from build123d import *

# Parameters (mm, degrees)
BOX_W                = 35
BOX_H                = 35
BOX_DEPTH            = 18
BOX001_W             = 1.5217
BOX001_H             = 35
BOX001_DEPTH         = 16.5
BOX002_W             = 1.5217
BOX002_H             = 35
BOX002_DEPTH         = 16.5
BOX003_W             = 1.5217
BOX003_H             = 35
BOX003_DEPTH         = 16.5
BOX004_W             = 1.5217
BOX004_H             = 35
BOX004_DEPTH         = 16.5
BOX005_W             = 7.6087
BOX005_H             = 35
BOX005_DEPTH         = 16.5
BOX006_W             = 1.5217
BOX006_H             = 35
BOX006_DEPTH         = 16.5
BOX007_W             = 1.5217
BOX007_H             = 35
BOX007_DEPTH         = 16.5
BOX008_W             = 1.5217
BOX008_H             = 35
BOX008_DEPTH         = 16.5
BOX009_W             = 1.5217
BOX009_H             = 35
BOX009_DEPTH         = 16.5
BODY_PLACEMENT_ANGLE = 90


with BuildPart() as part:
    # Box → Box (join)
    with BuildSketch(Plane(origin=(-17.5, -17.5, 0), x_dir=(1, 0, 0), z_dir=(0, 0, 1))):
        with Locations((17.5, 17.5)):
            Rectangle(BOX_W, BOX_H)
    extrude(amount=BOX_DEPTH)

    # Box001 → Box001 (cut)
    with BuildSketch(Plane(origin=(-15.978, -17.5, 1.5), x_dir=(1, 0, 0), z_dir=(0, 0, 1))):
        with Locations((0.76085, 17.5)):
            Rectangle(BOX001_W, BOX001_H)
    extrude(amount=BOX001_DEPTH, mode=Mode.SUBTRACT)

    # Box002 → Box002 (cut)
    with BuildSketch(Plane(origin=(-12.9347, -17.5, 1.5), x_dir=(1, 0, 0), z_dir=(0, 0, 1))):
        with Locations((0.76085, 17.5)):
            Rectangle(BOX002_W, BOX002_H)
    extrude(amount=BOX002_DEPTH, mode=Mode.SUBTRACT)

    # Box003 → Box003 (cut)
    with BuildSketch(Plane(origin=(-9.891304, -17.5, 1.5), x_dir=(1, 0, 0), z_dir=(0, 0, 1))):
        with Locations((0.76085, 17.5)):
            Rectangle(BOX003_W, BOX003_H)
    extrude(amount=BOX003_DEPTH, mode=Mode.SUBTRACT)

    # Box004 → Box004 (cut)
    with BuildSketch(Plane(origin=(-6.84782, -17.5, 1.5), x_dir=(1, 0, 0), z_dir=(0, 0, 1))):
        with Locations((0.76085, 17.5)):
            Rectangle(BOX004_W, BOX004_H)
    extrude(amount=BOX004_DEPTH, mode=Mode.SUBTRACT)

    # Box005 → Box005 (cut)
    with BuildSketch(Plane(origin=(-3.80434, -17.5, 1.5), x_dir=(1, 0, 0), z_dir=(0, 0, 1))):
        with Locations((3.80435, 17.5)):
            Rectangle(BOX005_W, BOX005_H)
    extrude(amount=BOX005_DEPTH, mode=Mode.SUBTRACT)

    # Box006 → Box006 (cut)
    with BuildSketch(Plane(origin=(5.326088, -17.5, 1.5), x_dir=(1, 0, 0), z_dir=(0, 0, 1))):
        with Locations((0.76085, 17.5)):
            Rectangle(BOX006_W, BOX006_H)
    extrude(amount=BOX006_DEPTH, mode=Mode.SUBTRACT)

    # Box007 → Box007 (cut)
    with BuildSketch(Plane(origin=(8.369566, -17.5, 1.5), x_dir=(1, 0, 0), z_dir=(0, 0, 1))):
        with Locations((0.76085, 17.5)):
            Rectangle(BOX007_W, BOX007_H)
    extrude(amount=BOX007_DEPTH, mode=Mode.SUBTRACT)

    # Box008 → Box008 (cut)
    with BuildSketch(Plane(origin=(11.407644, -17.5, 1.5), x_dir=(1, 0, 0), z_dir=(0, 0, 1))):
        with Locations((0.76085, 17.5)):
            Rectangle(BOX008_W, BOX008_H)
    extrude(amount=BOX008_DEPTH, mode=Mode.SUBTRACT)

    # Box009 → Box009 (cut)
    with BuildSketch(Plane(origin=(14.456521, -17.5, 1.5), x_dir=(1, 0, 0), z_dir=(0, 0, 1))):
        with Locations((0.76085, 17.5)):
            Rectangle(BOX009_W, BOX009_H)
    extrude(amount=BOX009_DEPTH, mode=Mode.SUBTRACT)


with BuildPart() as part_1:
    # Body placement: moved
    add(part.part.moved(Location((0, 0, 0.05))).rotate(Axis((0, 0, 0.05), (0, 0, 1)), BODY_PLACEMENT_ANGLE))


solid = part_1.part
Design review of the part built by this model. Coordinates are the model's own, in mm. A direction names the side the tool comes from. Give positions to 0.01 mm unless a question says otherwise; leave off trailing zeros. Order: outer loops, then holes, each group sorted by start corner. A loop starts at its lowest first (then second) coordinate and runs counter-clockwise, first axis right, second up.
1. Mouldability with a two-part tool opening along Y and no side actions: class faces 3 (the flat face through (0, 5, 18.05)), 4 (the flat face through (0, -12, 1.55)), 5 (the flat face through (0, -11.413, 10)), 6 (the flat face through (0, -17.5, 9)) as +Y half, -Y half, draft (parallel to the pull), parting line (faces both ways), or undercut.
Solution:
face 3: draft
face 4: undercut
face 5: undercut
face 6: -Y half
2. To check wall thickness, follow L1, parallel to Z at x = -12, y = -15.5. State the ranges of the line that lie inside material, in increasing order.
Solution:
L1: z = 0.05 to 1.55
3. Add section B-B, the plane y = 9. State the section outline as (x, z) points, then the cut area to 3 significant figures.
Solution:
outline: (-17.5, 0.05) - (17.5, 0.05) - (17.5, 1.55) - (-17.5, 1.55) - close
area: 52.5 mm2
4. For pin 1 Ø1.2 at (x, y) = (1, 12.5) entering from +Z; pin 2 Ø6 at (x, y) = (6.5, 0.5) entering from +Z, all flat-tipped, find the tip position at first contact; note any pin that passes through.
Solution:
pin 1: stops at z = 18.05
pin 2: stops at z = 1.55
5. Tool access review of faces 1 (the flat face through (0, 0, 0.05)), 2 (the flat face through (0, 5.326, 10)): name each direction out of +Z, -Z, +X, -X, +Y, -Y from which nothing blocks a thin tool from reaching the whole face with its end or side.
Solution:
face 1: -Z, +X, -X, +Y, -Y
face 2: +Z, +X, -X
6. Add section A-A, the plane z = 4.5. State how many separate pieces and enclosed holes the cut face has, then the cut area to 3 significant figures.
Solution:
separate pieces: 10
enclosed holes: 0
area: 533 mm2
